Work out the finished part from the listing and answer in its coordinate system (mm). Face numbers are marked on the shaded views. A direction names the side the tool comes from. Coordinates: 2 decimals unless noted, no trailing zeros. Write each loop counter-clockwise with the first axis right and the second up, starting at its lowest first coordinate (ties: lowest second). Pieces come first, ordered by that corner, then holes. Notation, with made-up numbers: (-37, 13.25) -> (1, 13.25) arc R18 cw to (1, 20.25) -> close; hole circle Ø3 at (-33.75, 50.5). An arc over 180 degrees is marked (long way). Write each question's results on one line, items separated by ' | '. Start each with the question number.
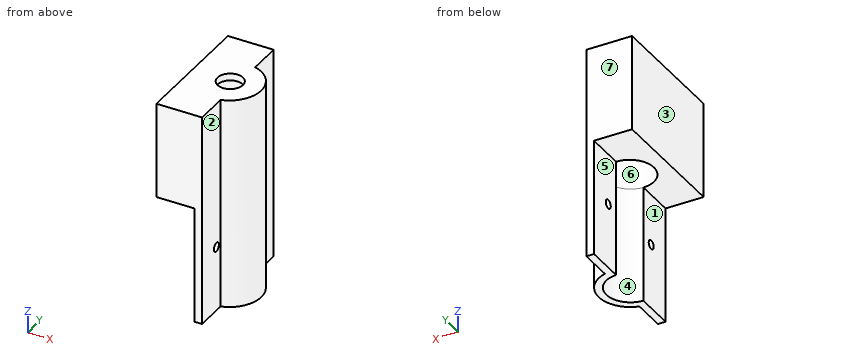
from build123d import *

# Parameters (mm, degrees)
F1_DEPTH  = 16
F2_R      = 9.5
F3_DEPTH  = 35
F5_DEPTH  = 40
F6_DEPTH  = 45.7
F7_W      = 50
F7_H      = 37.8
F8_DEPTH  = 15
F9_R      = 9.5
F10_DEPTH = 35
F11_R     = 5
F12_DEPTH = 25
F13_R     = 1.75
F14_DEPTH = 5


with BuildPart() as f1:
    # F0 (on Right) → F1 (new body)
    with BuildSketch(Plane.YZ):
        Polygon((-25, 0), (0, 0), (25, 0), (25, 38), (-25, 38), align=None)
    extrude(amount=F1_DEPTH)

    # F2 (on face) → F3 (cut)
    with BuildSketch(Plane(origin=(0, 0, 0), x_dir=(1, 0, 0), z_dir=(0, 0, -1))):
        with Locations((-0.3, 0)):
            Circle(F2_R)
    extrude(amount=-F3_DEPTH, mode=Mode.SUBTRACT)

    # F4 (on face) → F5 (cut)
    with BuildSketch(Plane(origin=(0, 0, 0), x_dir=(1, 0, 0), z_dir=(0, 0, -1))):
        with BuildLine():
            Line((16, 25), (3, 25))
            Line((3, 25), (3, 12.0565332544))
            ThreePointArc((3, 12.0565332544), (12.1999997646, 0), (3, -12.0565332544))
            Line((3, -12.0565332544), (3, -25))
            Line((3, -25), (16, -25))
            Line((16, -25), (16, 25))
        make_face()
    extrude(amount=-F5_DEPTH, mode=Mode.SUBTRACT)

    # F6 (add): a face of the model
    f6_faces = [f1.faces().sort_by_distance(p)[0] for p in [
        (0.514668825, -17.2476309882, 0),
    ]]
    extrude(f6_faces, amount=F6_DEPTH)

    # F7 (on face) → F8 (join)
    with BuildSketch(Plane(origin=(0, 0, 0), x_dir=(0, -1, 0), z_dir=(-1, 0, 0))):
        with Locations((0, 19.1)):
            Rectangle(F7_W, F7_H)
    extrude(amount=F8_DEPTH)

    # F9 (on face) → F10 (cut)
    with BuildSketch(Plane(origin=(0, 0, 0.2), x_dir=(1, 0, 0), z_dir=(0, 0, -1))):
        Circle(F9_R)
    extrude(amount=-F10_DEPTH, mode=Mode.SUBTRACT)

    # F11 (on face) → F12 (cut)
    with BuildSketch(Plane.XY.offset(38)):
        Circle(F11_R)
    extrude(amount=-F12_DEPTH, mode=Mode.SUBTRACT)

    # F13 (on face) → F14 (cut)
    with BuildSketch(Plane(origin=(0, 0, 0), x_dir=(0, -1, 0), z_dir=(-1, 0, 0))):
        with Locations((-15, -20)):
            Circle(F13_R)
        with Locations((15, -20)):
            Circle(F13_R)
    extrude(amount=-F14_DEPTH, mode=Mode.SUBTRACT)


solid = f1.part
1. Find the intervals of material crossed by L1, parallel to Y at x = 0, z = 36.2; L2, parallel to X at y = 0, z = 22; L3, parallel to Z at x = 1.4, y = -15, in increasing order.
2. For the marked faces 1, 2 and 3, determine the directions among +Z, -Z, +X, -X, +Y, -Y from which every point of the face is accessible in a straight line to the end or side of a thin tool.
3. Find section D-D on y = -19.5. Give the vertices of the cut face in (x, z).
4. Determine the mould class of the marked faces 4, 5, 6 and 7 for opening direction Y: pulls with the +Y half, pulls with the -Y half, needs draft (parallel to the pull), parting line crosses it, or undercut.
5. Find section C-C on z = 22.5. Give the vertices of the cut face in (x, y).
6. Given pin 1 Ø5 at (y, z) = (-6, -25) entering from +X; pin 2 Ø12.5 at (y, z) = (15, -28.5) entering from -X; pin 3 Ø7.5 at (x, y) = (-5, 7) entering from -Z; pin 4 Ø12 at (x, y) = (0.5, 0) entering from +Z, each flat-ended and moving along its own axis, determine where each tip first touches the part or whether it passes through.
7. Find section A-A on y = 0. Give the vertices of the cut face in (x, z), and give its area (3 significant figures).
Ans:
1) L1: y = -25 to -5, 5 to 25 | L2: x = -15 to -9.5, 9.5 to 12.2 | L3: z = -45.7 to -21.75, -18.25 to 38
2) face 1: -Z, -X, +Y, -Y | face 2: +Z, -Z, +X, -Y | face 3: +Z, -Z, -X, +Y, -Y
3) outline: (-15, 0.2) -> (0, 0.2) -> (0, -45.7) -> (3, -45.7) -> (3, 38) -> (-15, 38) -> close
4) face 4: undercut | face 5: needs draft | face 6: undercut | face 7: pulls with the +Y half
5) outline: (-15, -25) -> (3, -25) -> (3, -12.06) arc R12.5 ccw to (3, 12.06) -> (3, 25) -> (-15, 25) -> close; hole circle Ø19 at (0, 0)
6) pin 1: stops at x = 11.7 | pin 2: stops at x = 0 | pin 3: stops at z = 0.2 | pin 4: stops at z = 38
7) outline: (-15, 0.2) -> (-9.5, 0.2) -> (-9.5, 35.2) -> (-5, 35.2) -> (-5, 38) -> (-15, 38) -> close; (5, 35.2) -> (9.5, 35.2) -> (9.5, 0.2) -> (9.2, 0.2) -> (9.2, -45.7) -> (12.2, -45.7) -> (12.2, 38) -> (5, 38) -> close | area: 473 mm²
